```python
from build123d import *

# Parameters (mm, degrees)
EXTRUDE_1_DEPTH     = 15
SHELL_1_T           = -3
CUT_EXTRUDE_1_DEPTH = 676.11573082
SKETCH_4_R          = 2.1
CUT_EXTRUDE_2_DEPTH = 675.121836169
SKETCH_5_R          = 2.1
CUT_EXTRUDE_3_DEPTH = 3


with BuildPart() as part:
    # 草图1 → 凸台-拉伸1 (new, symmetric)
    with BuildSketch(Plane.XY):
        with BuildLine():
            Line((0, 0), (0, 100))
            ThreePointArc((0, 100), (56.25, 156.25), (112.5, 100))
            Line((112.5, 100), (112.5, -665))
            Line((112.5, -665), (92.5, -665))
            Line((92.5, -665), (92.5, 100))
            ThreePointArc((92.5, 100), (56.25, 136.25), (20, 100))
            Line((20, 100), (20, 0))
            Line((20, 0), (0, 0))
        make_face()
    extrude(amount=EXTRUDE_1_DEPTH, both=True)

    # 抽壳1
    shell_1_openings = [part.faces().sort_by_distance(p)[0] for p in [
        (102.5, -665, 0),
        (10, 0, 0),
    ]]
    offset(amount=SHELL_1_T, openings=shell_1_openings, kind=Kind.INTERSECTION)

    # 草图3 → 切除-拉伸1 (cut, through all)
    with BuildSketch(Plane.XY.offset(15)):
        Polygon((12, 0), (20, 17), (20, 0), align=None)
        Polygon((92.5, -665), (92.5, -648), (100.5, -665), align=None)
    extrude(amount=-CUT_EXTRUDE_1_DEPTH, mode=Mode.SUBTRACT)

    # 草图4 → 切除-拉伸2 (cut, through all)
    with BuildSketch(Plane.ZY.offset(-109.5)):
        with Locations(Location((-5, -657, 0), (0, 0, 270))):
            Circle(SKETCH_4_R)
        with Locations(Location((5, -657, 0), (0, 0, 270))):
            Circle(SKETCH_4_R)
    extrude(amount=-CUT_EXTRUDE_2_DEPTH, mode=Mode.SUBTRACT)

    # 草图5 → 切除-拉伸3 (cut)
    with BuildSketch(Plane.ZY):
        with Locations((-5, 8)):
            Circle(SKETCH_5_R)
        with Locations((5, 8)):
            Circle(SKETCH_5_R)
    extrude(amount=-CUT_EXTRUDE_3_DEPTH, mode=Mode.SUBTRACT)


solid = part.part
```
For this review, take the finished solid that the model builds, in its own axes (mm). A direction names the side the tool comes from. Coordinates: 2 decimals unless noted, no trailing zeros. Loops run counter-clockwise (first coordinate to the right, second up) from the corner with the lowest first, then second, coordinate; pieces in that order, holes last. Notation, with made-up numbers: (-20.75, -6.5) - (36.25, -6.5) arc R12 cw to (36.25, 12.5) - close; hole circle Ø9 at (-28, -1.5). An arc over 180 degrees is marked (long way). Use one line per item in the form item = value. Start each with the question number.
1) Draft analysis for pull direction Z (two halves, no side actions). For faces 5 (the face through (3, 49, 0)), 6 (the face through (94, -192, 15)), 7 (the face through (92.5, -279, 0)), state which applies: released by +Z, released by -Z, zero draft, split by the parting line, or undercut.
2) To check wall thickness, follow probe 1 along X at (y, z) = (92, 10.5); probe 2 along Z at (x, y) = (110.7, -657); probe 3 along X at (y, z) = (-319, -1.5). State the ranges of each line that lie inside material, in increasing order. Write a range as from..to.
3) Take a section at A-A (y = 69). State the section outline as (x, z) points.
4) Take a section at C-C (y = -137). State the section outline as (x, z) points.
5) Take a section at B-B (x = 56.25). State the section outline as (y, z) points, plus the area to 3 significant figures.
6) For faces 1 (the face through (20, 59, 0)), 2 (the face through (17, 56, 0)), 3 (the face through (112.5, -277, 0)), 4 (the face through (57.11, 139.24, 0.17)), list the 3-axis set-ups (+Z, -Z, +X, -X, +Y, -Y) from which the entire face can be reached by the end or side of a thin tool; tool diameter is ignored.
7) For pin 1 (8 mm diameter, centred on x = 43.5, z = 3.5, fed in from -Y); pin 2 (5 mm diameter, centred on y = -345.5, z = -10, fed in from -X); pin 3 (6 mm diameter, centred on x = 3, z = 0, fed in from -Y), all flat-tipped, find the tip position at first contact; note any pin that passes through.
From the geometry:
q1.face_5 = undercut
q1.face_6 = released by +Z
q1.face_7 = zero draft
q2.probe_1 = 0..3, 17..20, 92.5..95.5, 109.5..112.5
q2.probe_2 = -15..-7.1, -2.9..2.9, 7.1..15
q2.probe_3 = 92.5..95.5, 109.5..112.5
q3.outline = (0, -15) - (20, -15) - (20, 15) - (0, 15) - close; (92.5, -15) - (112.5, -15) - (112.5, 15) - (92.5, 15) - close; hole (3, -12) - (17, -12) - (17, 12) - (3, 12) - close; hole (95.5, -12) - (109.5, -12) - (109.5, 12) - (95.5, 12) - close
q4.outline = (92.5, -15) - (112.5, -15) - (112.5, 15) - (92.5, 15) - close; hole (95.5, -12) - (109.5, -12) - (109.5, 12) - (95.5, 12) - close
q5.outline = (136.25, -15) - (156.25, -15) - (156.25, 15) - (136.25, 15) - close; hole (139.25, -12) - (153.25, -12) - (153.25, 12) - (139.25, 12) - close
q5.area = 264 mm2
q6.face_1 = +Z, -Z, -Y
q6.face_2 = -Y
q6.face_3 = +Z, -Z, +X, +Y, -Y
q6.face_4 = none
q7.pin_1 = 132.15
q7.pin_2 = 92.5
q7.pin_3 = 0
